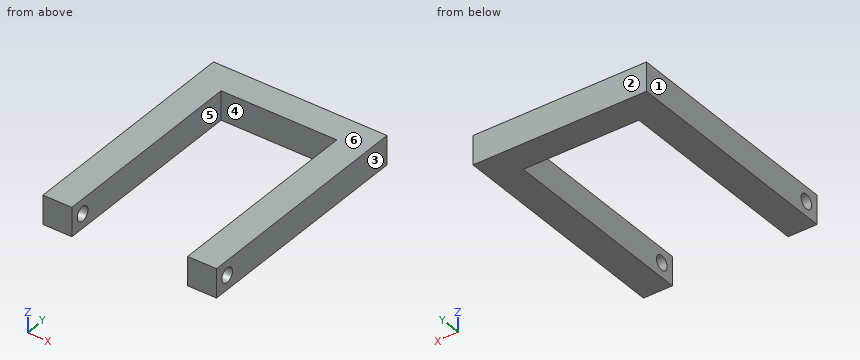
```python
from build123d import *

# Parameters (mm, degrees)
F1_DEPTH = 10
F2_R     = 5
F3_DEPTH = 60


with BuildPart() as f1:
    # F0 (on Top) → F1 (new body, symmetric)
    with BuildSketch(Plane.XY):
        Polygon((40, -80), (60, -80), (60, 80), (-60, 80), (-60, -80), (-40, -80), (-40, -60), (-40, 60), (40, 60), (40, -60), align=None)
    extrude(amount=F1_DEPTH, both=True)

    # F2 (on Right) → F3 (cut, symmetric)
    with BuildSketch(Plane.YZ):
        with Locations((-70, 0)):
            Circle(F2_R)
    extrude(amount=F3_DEPTH, both=True, mode=Mode.SUBTRACT)


solid = f1.part
```
Model file for the job. Use its own axes, mm. Face numbers are marked on the shaded views. A direction names the side the tool comes from. Coordinates: 2 decimals unless noted, no trailing zeros. Order: outer loops, then holes, each group sorted by start corner. A loop starts at its lowest first (then second) coordinate and runs counter-clockwise, first axis right, second up. Notation, with made-up numbers: (83.25, 46.25) -> (136.25, 46.25) arc R30 ccw to (136.25, 80.25) -> close; hole circle Ø5 at (-38, -0.5). An arc over 180 degrees is marked (long way). Return JSON: item names as keys, results as strings.
Item 1: Slice it at B-B (z = 0). Write the cut outline in (x, y).
Model answer:
{"outline": "(-60, -80) -> (-40, -80) -> (-40, -75) -> (-60, -75) -> close; (-60, -65) -> (-40, -65) -> (-40, 60) -> (40, 60) -> (40, -65) -> (60, -65) -> (60, 80) -> (-60, 80) -> close; (40, -80) -> (60, -80) -> (60, -75) -> (40, -75) -> close"}
Item 2: Mould opens along X. For the marked faces 1, 2, 3 and 4 say: pulls with the +X half, pulls with the -X half, needs draft (parallel to the pull), parting line crosses it, or undercut.
Model answer:
{"face 1": "pulls with the -X half", "face 2": "needs draft", "face 3": "pulls with the +X half", "face 4": "undercut"}
Item 3: Slice it at D-D (x = -2.5). Write the cut outline in (y, z).
Model answer:
{"outline": "(60, -10) -> (80, -10) -> (80, 10) -> (60, 10) -> close"}
Item 4: Wall check: line 1 along X through (y, z) = (16, 9); line 2 along Z through (x, y) = (-44.75, -70); line 3 along Y through (x, z) = (23.5, -6.5). Give the ranges that are in metal, low to high. Write a range as from..to.
Model answer:
{"line 1": "x = -60..-40, 40..60", "line 2": "z = -10..-5, 5..10", "line 3": "y = 60..80"}
Item 5: Slice it at C-C (x = -45.5). Write the cut outline in (y, z).
Model answer:
{"outline": "(-80, -10) -> (80, -10) -> (80, 10) -> (-80, 10) -> close; hole circle Ø10 at (-70, 0)"}
Item 6: 3-axis set-ups, long thin cutter, end or side, ignore diameter. For the marked faces 5 and 6: which of +Z, -Z, +X, -X, +Y, -Y reach the whole face in a straight line?
Model answer:
{"face 5": "+Z, -Z, -Y", "face 6": "+Z, +X, -X, +Y, -Y"}
Item 7: Slice it at A-A (y = -60). Write the cut outline in (x, z), then the cut area to 3 significant figures.
Model answer:
{"outline": "(-60, -10) -> (-40, -10) -> (-40, 10) -> (-60, 10) -> close; (40, -10) -> (60, -10) -> (60, 10) -> (40, 10) -> close", "area": "800 mm²"}
Item 8: Pin check, flat tip, straight feed: P1, Ø10, axis at x = 11, z = 2, coming from the -Y side. Stop position of the tip, or through.
Model answer:
{"P1": "stops at y = 60"}
